from build123d import *

# Parameters (mm, degrees)
F2_R     = 7.709402
F3_DEPTH = 88.9
F4_R     = 5.08
F5_R     = 5.08


with BuildPart() as f1:
    # F0 (on Front) → F1 (revolve)
    with BuildSketch(Plane.XZ):
        Polygon((0, 63.5), (0, 0), (45.4152, 34.417), (45.4152, 50.1904), (13.868312, 50.1904), (13.868312, 63.5), align=None)
    revolve(axis=Axis((0, 0, 31.75), (0, 0, -1)))

    # F2 (on face) → F3 (cut)
    with BuildSketch(Plane.XY.offset(63.5)):
        Circle(F2_R)
    extrude(amount=-F3_DEPTH, mode=Mode.SUBTRACT)

    # F4
    f4_edges = [f1.edges().sort_by_distance(p)[0] for p in [
        (-45.4152, 0, 50.1904),
        (-13.868312, 0, 50.1904),
    ]]
    fillet(f4_edges, radius=F4_R)

    # F5
    f5_edges = [f1.edges().sort_by_distance(p)[0] for p in [
        (-7.709402, 0, 5.842416),
        (26.562301, 0, 20.129708),
        (-45.4152, 0, 34.417),
    ]]
    fillet(f5_edges, radius=F5_R)


solid = f1.part
Build history of the part. All positions in model axes, mm. A direction names the side the tool comes from. Give positions to 0.01 mm unless a question says otherwise; leave off trailing zeros. Order: outer loops, then holes, each group sorted by start corner. A loop starts at its lowest first (then second) coordinate and runs counter-clockwise, first axis right, second up. Notation, with made-up numbers: M -34,21.25 L 5,21.25 A19 ccw 5,50.25 Z; hole C 76.25,78 d9. An arc over 180 degrees is marked long. Put each result on its own line as item: value.
Item 1: 3-axis set-ups, long thin cutter, end or side, ignore diameter. For faces 1 (the flat face through (8.4, 17.4, 50.19)), 2 (the conical face through (16.24, 6.73, 13.32)): which of +Z, -Z, +X, -X, +Y, -Y reach the whole face in a straight line?
From the geometry:
face 1: +Z
face 2: -Z
Item 2: Slice it at B-B, the plane z = 53. Write the cut outline in (x, y), plus the area to 3 significant figures.
From the geometry:
outline: C 0,0 d28.81; hole C 0,0 d15.42
area: 465 mm2
Item 3: Two-plate mould, pull along X, no slides. Class faces 3 (the cylindrical face through (43.32, -13.64, 41.08)), 4 (the cylindrical face through (7.35, 2.32, 40.12)), 5 (the flat face through (6, 6, 63.5)): +X half, -X half, draft (parallel to the pull), parting line (faces both ways), or undercut.
From the geometry:
face 3: parting line
face 4: undercut
face 5: draft
Item 4: Probe line 1 (X direction, y = 0, z = 39.5); line 2 (Z direction, x = -5, y = -11.5); line 3 (Y direction, x = -6, z = 32). List the from-to ranges inside material, lowest first. Write a range as [from, to].
From the geometry:
line 1: x = [-45.42, -7.71], [7.71, 45.42]
line 2: z = [10.99, 63.5]
line 3: y = [-41.8, -4.84], [4.84, 41.8]
Item 5: Slice it at A-A, the plane z = 22. Write the cut outline in (x, y), plus the area to 3 significant figures.
From the geometry:
outline: C 0,0 d58.06; hole C 0,0 d15.42
area: 2,460 mm2
Item 6: Flat gauge pins, fed straight in: pin 1 Ø5 at (x, y) = (35, -6) entering from -Z; pin 2 Ø5 at (x, y) = (-9.5, -1.5) entering from -Z; pin 3 Ø1 at (x, z) = (-15.5, 27.5) entering from +Y; pin 4 Ø2 at (y, z) = (27.5, 52.5) entering from +X. Where does each tip first touch, or does it go through?
From the geometry:
pin 1: stops at z = 25.02
pin 2: stops at z = 11.03
pin 3: stops at y = 33.57
pin 4: passes through
